Geometry check sheet. Reference: the model listing, model coordinates, mm. A direction names the side the tool comes from. Give positions to 0.01 mm unless a question says otherwise; leave off trailing zeros. Loops run counter-clockwise (first coordinate to the right, second up) from the corner with the lowest first, then second, coordinate; pieces in that order, holes last. Notation, with made-up numbers: (-1.5, 45.25) -> (55.5, 45.25) arc R20 cw to (55.5, 78.25) -> close; hole circle Ø7 at (88.25, 28). An arc over 180 degrees is marked (long way). Answer as a JSON object with one key per item and string values.
from build123d import *

# Parameters (mm, degrees)
SKETCH1_W           = 190
SKETCH1_H           = 150
BOSS_EXTRUDE1_DEPTH = 60.5
SKETCH3_W           = 60.5
SKETCH3_H           = 150
BOSS_EXTRUDE2_DEPTH = 25
SKETCH4_W           = 450
SKETCH4_H           = 650
BOSS_EXTRUDE3_DEPTH = 39.5
BOSS_EXTRUDE4_DEPTH = 650


with BuildPart() as part:
    # Sketch1 → Boss-Extrude1 (new body)
    with BuildSketch(Plane.XY):
        with Locations((0, 250)):
            Rectangle(SKETCH1_W, SKETCH1_H)
        Polygon((-95, -175), (-95, 175), (-95, 325), (-330, 325), (-330, -325), (95, -325), (95, -175), align=None)
    extrude(amount=BOSS_EXTRUDE1_DEPTH)

    # Sketch3 → Boss-Extrude2 (add)
    with BuildSketch(Plane(origin=(95, 0, 0), x_dir=(0, 0, -1), z_dir=(1, 0, 0))):
        Polygon((-70.5, -325), (0, -325), (0, 175), (-60.5, 175), (-60.5, 325), (-70.5, 325), align=None)
        with Locations((-30.25, 250)):
            Rectangle(SKETCH3_W, SKETCH3_H)
    extrude(amount=BOSS_EXTRUDE2_DEPTH)

    # Sketch4 → Boss-Extrude3 (add)
    with BuildSketch(Plane(origin=(0, 0, 0), x_dir=(-1, 0, 0), z_dir=(0, 0, -1))):
        with Locations((105, 0)):
            Rectangle(SKETCH4_W, SKETCH4_H)
    extrude(amount=BOSS_EXTRUDE3_DEPTH)

    # Sketch8 → Boss-Extrude4 (add)
    with BuildSketch(Plane(origin=(0, 325, 0), x_dir=(1, 0, 0), z_dir=(0, 1, 0))):
        Polygon((-330, -60.5), (-700, 39.5), (-330, 39.5), align=None)
    extrude(amount=-BOSS_EXTRUDE4_DEPTH)


solid = part.part
1) Section check D-D on y = 247. Record the cut outline in (x, z).
Geometry check:
{"outline": "(-700, -39.5) -> (120, -39.5) -> (120, 70.5) -> (95, 70.5) -> (95, 60.5) -> (-330, 60.5) -> close"}
2) Tool access check on faces 1 (the face through (-168, 5, 60.5)), 2 (the face through (95, 5, 36)), 3 (the face through (120, -5, 16)). Record the directions out of +Z, -Z, +X, -X, +Y, -Y that give a thin tool (end or side, any length) a straight path to the whole face; none if there is none.
Geometry check:
{"face 1": "+Z, -X, +Y, -Y", "face 2": "+Z", "face 3": "+Z, -Z, +X, +Y, -Y"}
3) Material ranges on line 1 along Y through (x, z) = (-77.5, 18.5); line 2 along Z through (x, y) = (9, 183.5); line 3 along Z through (x, y) = (-31.5, 44), recorded low to high. Write a range as from..to.
Geometry check:
{"line 1": "y = -325..-175, 175..325", "line 2": "z = -39.5..60.5", "line 3": "z = -39.5..0"}
4) Section check A-A on z = 42. Record the cut outline in (x, y), plus the area to 3 significant figures.
Geometry check:
{"outline": "(-398.45, -325) -> (120, -325) -> (120, 325) -> (-398.45, 325) -> close; hole (-95, -175) -> (95, -175) -> (95, 175) -> (-95, 175) -> close", "area": "270,000 mm2"}
5) Draft check along Y on faces 4 (the face through (1, 2, 0)), 5 (the face through (-193, 325, 3)), 6 (the face through (-512.41, 4.55, 11.2)). Enter one of: pulls with the +Y half, pulls with the -Y half, needs draft (parallel to the pull), parting line crosses it, or undercut.
Geometry check:
{"face 4": "undercut", "face 5": "pulls with the +Y half", "face 6": "needs draft"}
6) Depth check by flat-ended pin: P1, Ø3, axis at x = -82.5, y = -146.5, coming from the +Z side; P2, Ø10, axis at x = -375.5, y = -95.5, coming from the +Z side. Enter the tip coordinate at first touch or a pass-through.
Geometry check:
{"P1": "stops at z = 0", "P2": "stops at z = 49.55"}
7) Section check C-C on y = -14.5. Record the cut outline in (x, z), plus the area to 3 significant figures.
Geometry check:
{"outline": "(-700, -39.5) -> (120, -39.5) -> (120, 70.5) -> (95, 70.5) -> (95, 0) -> (-95, 0) -> (-95, 60.5) -> (-330, 60.5) -> close", "area": "52,300 mm2"}
8) Section check B-B on x = -49. Record the cut outline in (y, z).
Geometry check:
{"outline": "(-325, -39.5) -> (325, -39.5) -> (325, 60.5) -> (175, 60.5) -> (175, 0) -> (-175, 0) -> (-175, 60.5) -> (-325, 60.5) -> close"}
